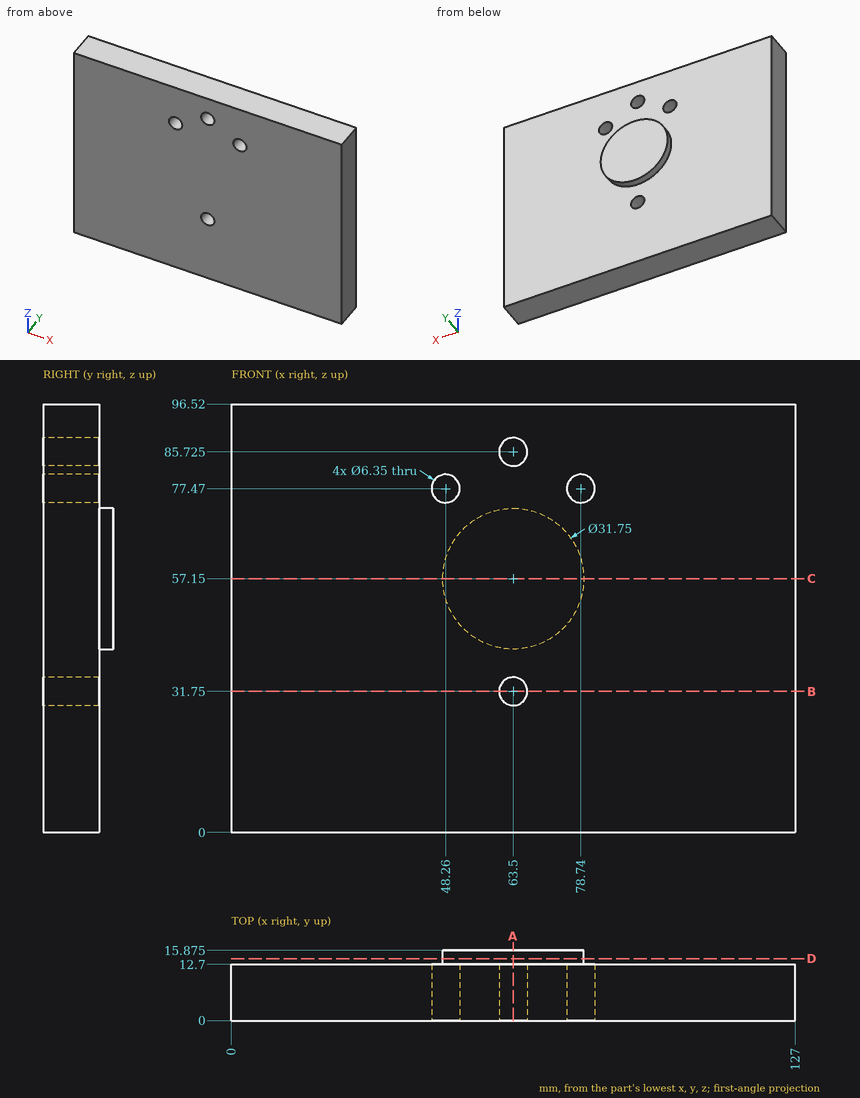
Print and shaded views of the part. All mm, measured from the part's lowest x, y and z. Coordinates: 2 decimals unless noted, no trailing zeros. Loops run counter-clockwise (first coordinate to the right, second up) from the corner with the lowest first, then second, coordinate; pieces in that order, holes last. Notation, with made-up numbers: M 26,42 L 44,42 A25 ccw 44,67 Z; hole C 66.25,62 d5. An arc over 180 degrees is marked long. Use a Markdown table: item, result. Add a question column.
Q1. Cut at D-D (y = 14). Write the cut outline in (x, z) (3 decimals).
Q2. Cut at C-C (z = 57.15). Write the cut outline in (x, y) (3 decimals).
Q3. Pin check, flat tips, straight feed: P1, Ø5.5, axis at x = 48.26, z = 77.47, coming from the +Y side; P2, Ø1.5, axis at x = 81.5, z = 73.5, coming from the +Y side. Stop position of each tip, or through.
Q4. Probe L1, parallel to X at y = 8, z = 77.47 (3 decimals); L2, parallel to Z at x = 63.5, y = 9 (3 decimals); L3, parallel to Z at x = 78.5, y = 7.25. List the from-to ranges inside material, lowest first.
Q5. Cut at B-B (z = 31.75). Write the cut outline in (x, y) (3 decimals).
Q6. Cut at A-A (x = 63.5). Write the cut outline in (y, z) (3 decimals), and give its area (3 significant figures).
Worked out:
| question | item | result |
|---|---|---|
| 1 | outline | C 63.5,57.15 d31.75 |
| 2 | outline | M 0,0 L 127,0 L 127,12.7 L 79.375,12.7 L 79.375,15.875 L 47.625,15.875 L 47.625,12.7 L 0,12.7 Z |
| 3 | P1 | passes through |
| 3 | P2 | stops at y = 12.7 |
| 4 | L1 | x = 0 to 45.085, 51.435 to 75.565, 81.915 to 127 |
| 4 | L2 | z = 0 to 28.575, 34.925 to 82.55, 88.9 to 96.52 |
| 4 | L3 | z = 0 to 74.3, 80.64 to 96.52 |
| 5 | outline | M 0,0 L 60.325,0 L 60.325,12.7 L 0,12.7 Z; M 66.675,0 L 127,0 L 127,12.7 L 66.675,12.7 Z |
| 6 | outline | M 0,0 L 12.7,0 L 12.7,28.575 L 0,28.575 Z; M 0,34.925 L 12.7,34.925 L 12.7,41.275 L 15.875,41.275 L 15.875,73.025 L 12.7,73.025 L 12.7,82.55 L 0,82.55 Z; M 0,88.9 L 12.7,88.9 L 12.7,96.52 L 0,96.52 Z |
| 6 | area | 1,170 mm2 |
